Check sheet for the modelled part. Datum: model origin and axes. Units: mm. A direction names the side the tool comes from. Round coordinates to 2 decimals unless told otherwise and drop trailing zeros. Loops run counter-clockwise (first coordinate to the right, second up) from the corner with the lowest first, then second, coordinate; pieces in that order, holes last. Notation, with made-up numbers: M -39,81.5 L 8,81.5 A25 ccw 8,116.5 Z; hole C -32.5,89.5 d7. An arc over 180 degrees is marked long. One line per question, with ' | ' between items. Start each with the question number.
(1) Section check C-C (x = 842). Record the boundary of the cut face in (y, z) (3 decimals).
(2) Section check D-D (y = 13). Record the boundary of the cut face in (x, z) (3 decimals), and give its area (3 significant figures).
(3) Section check B-B (z = -21.5). Record the boundary of the cut face in (x, y).
(4) Draft check along X on faces 3 (the face through (863.31, 22.94, -11.75)), 4 (the face through (847.541, -3.072, -0.905)), 5 (the face through (821.38, 8, 1)). Enter one of: +X half, -X half, draft (parallel to the pull), parting line (faces both ways), or undercut.
(5) Section check A-A (z = -12.7). Record the boundary of the cut face in (x, y), and give its area (3 significant figures).
(6) Go/stop test with flat-tipped pins: P1, Ø15, axis at x = 837, y = 12.5, coming from the -Z side; P2, Ø4, axis at x = 850.5, y = 3, coming from the -Z side. Record where each tip stops, or that it passes through.
(7) Thickness scan on probe 1 along Y at (x, z) = (839, -14.5); probe 2 along Z at (x, y) = (868.5, 13) (3 decimals); probe 3 along Z at (x, y) = (841, 22). Record the ranges inside material, lowest first. Write a range as [from, to].
(8) Tool access check on faces 1 (the face through (831.71, 22.94, -12.56)), 2 (the face through (847.541, 20.468, -0.955)). Record the directions out of +Z, -Z, +X, -X, +Y, -Y that give a thin tool (end or side, any length) a straight path to the whole face; none if there is none.
```python
from build123d import *

# Parameters (mm, degrees)
SKETCH1_W          = 889
SKETCH1_H          = 31.75
EXTRUDE1_DEPTH     = 28.575
EXTRUDE2_REACH     = 891
SKETCH2_W          = 25.4
SKETCH2_H          = 25.4
HOLE1_D            = 6.35
HOLE1_DEPTH        = 3.175
LPATTERN1_COUNT    = 35
LPATTERN1_PITCH    = 25.4
HOLE2_D            = 9.652
HOLE2_DEPTH        = 3.175
LPATTERN2_COUNT    = 12
LPATTERN2_PITCH    = 25.4
HOLE3_D            = 9.652
HOLE3_DEPTH        = 3.175
HOLE4_D            = 9.652
HOLE4_DEPTH        = 3.175
LPATTERN3_COUNT    = 12
LPATTERN3_PITCH    = 25.4
HOLE5_D            = 3.175
HOLE5_DEPTH        = 3.175
HOLE6_D            = 6.35
HOLE6_DEPTH        = 3.175
LPATTERN4_COUNT    = 35
LPATTERN4_PITCH    = 25.4
FILLET1_R          = 3.175
FILLET2_R          = 3.175
FILLET3_R          = 6.35
FILLET4_R          = 6.35
SKETCH16_W         = 145.760071232
SKETCH16_H         = 71.504803879
CUT_EXTRUDE2_DEPTH = 75
SKETCH17_W         = 473.628565651
SKETCH17_H         = 66.908943447
CUT_EXTRUDE3_DEPTH = 186
SKETCH18_W         = 383.094897193
SKETCH18_H         = 93.915816603
CUT_EXTRUDE4_DEPTH = 186
SKETCH19_W         = 44.323760151
SKETCH19_H         = 53.749642994
CUT_EXTRUDE5_DEPTH = 186


with BuildPart() as part:
    # Sketch1 → Extrude1 (new body)
    with BuildSketch(Plane.XY.offset(3.175)):
        with Locations((428.480011997, 8.672957166)):
            Rectangle(SKETCH1_W, SKETCH1_H)
    extrude(amount=-EXTRUDE1_DEPTH)

    # Sketch2 → Extrude2 (cut, up to next)
    with BuildSketch(Plane.ZY.offset(16.019988003), mode=Mode.PRIVATE) as extrude2_sk1:
        with Locations((-12.7, 8.672957166)):
            Rectangle(SKETCH2_W, SKETCH2_H)
    extrude2_tool1 = extrude(extrude2_sk1.sketch, amount=-EXTRUDE2_REACH, mode=Mode.PRIVATE) & part.part
    add(extrude2_tool1.solids().sort_by_distance((-16.019988, 8.672957, -12.7))[0], mode=Mode.SUBTRACT)

    # Hole1
    with Locations(Plane(origin=(0, 24.547957166, 0), x_dir=(-1, 0, 0), z_dir=(0, 1, 0))):
        with Locations((3.319988003, -12.7)):
            hole1 = Hole(HOLE1_D / 2, depth=HOLE1_DEPTH)

    # LPattern1: Hole1 ×35
    with Locations(*[(i * LPATTERN1_PITCH, 0, 0) for i in range(1, LPATTERN1_COUNT)]):
        add(hole1, mode=Mode.SUBTRACT)

    # Hole2
    with Locations(Plane.XY.offset(3.175)):
        with Locations((66.530011997, 10.577957166)):
            hole2 = Hole(HOLE2_D / 2, depth=HOLE2_DEPTH)

    # LPattern2: Hole2 ×12, 8 skipped
    with Locations(*[(i * LPATTERN2_PITCH, 0, 0) for i in range(1, LPATTERN2_COUNT) if i not in (2, 3, 4, 5, 6, 7, 8, 9)]):
        add(hole2, mode=Mode.SUBTRACT)

    # Hole3
    with Locations(Plane.XY.offset(3.175)):
        with Locations((428.480011997, 6.767957166)):
            Hole(HOLE3_D / 2, depth=HOLE3_DEPTH)

    # Hole4
    with Locations(Plane.XY.offset(3.175)):
        with Locations((511.030011997, 10.577957166)):
            hole4 = Hole(HOLE4_D / 2, depth=HOLE4_DEPTH)

    # LPattern3: Hole4 ×12, 8 skipped
    with Locations(*[(i * LPATTERN3_PITCH, 0, 0) for i in range(1, LPATTERN3_COUNT) if i not in (2, 3, 4, 5, 6, 7, 8, 9)]):
        add(hole4, mode=Mode.SUBTRACT)

    # Hole5
    with Locations(Plane.XY.offset(3.175)):
        with Locations((669.780011997, 8.672957166)):
            Hole(HOLE5_D / 2, depth=HOLE5_DEPTH)

    # Hole6
    with Locations(Plane(origin=(0, -4.027042834, 0), x_dir=(-1, 0, 0), z_dir=(0, 1, 0))):
        with Locations((3.319988003, -12.7)):
            hole6 = Hole(HOLE6_D / 2, depth=HOLE6_DEPTH)

    # LPattern4: Hole6 ×35
    with Locations(*[(i * LPATTERN4_PITCH, 0, 0) for i in range(1, LPATTERN4_COUNT)]):
        add(hole6, mode=Mode.SUBTRACT)

    # Fillet1
    fillet1_edges = [part.edges().sort_by_distance(p)[0] for p in [
        (428.480011997, 21.372957166, 0),
    ]]
    fillet(fillet1_edges, radius=FILLET1_R)

    # Fillet2
    fillet2_edges = [part.edges().sort_by_distance(p)[0] for p in [
        (428.480011997, -4.027042834, 0),
    ]]
    fillet(fillet2_edges, radius=FILLET2_R)

    # Fillet3
    fillet3_edges = [part.edges().sort_by_distance(p)[0] for p in [
        (428.480011997, -7.202042834, 3.175),
    ]]
    fillet(fillet3_edges, radius=FILLET3_R)

    # Fillet4
    fillet4_edges = [part.edges().sort_by_distance(p)[0] for p in [
        (428.480011997, 24.547957166, 3.175),
    ]]
    fillet(fillet4_edges, radius=FILLET4_R)

    # Sketch16 → Cut-Extrude2 (cut)
    with BuildSketch(Plane(origin=(0, 24.547957166, 0), x_dir=(1, 0, 0), z_dir=(0, 1, 0))):
        with Locations((40.099976381, -10.352401939)):
            Rectangle(SKETCH16_W, SKETCH16_H)
    extrude(amount=-CUT_EXTRUDE2_DEPTH, mode=Mode.SUBTRACT)

    # Sketch17 → Cut-Extrude3 (cut)
    with BuildSketch(Plane(origin=(0, 24.547957166, 0), x_dir=(1, 0, 0), z_dir=(0, 1, 0))):
        with Locations((288.165729172, -8.054471723)):
            Rectangle(SKETCH17_W, SKETCH17_H)
    extrude(amount=-CUT_EXTRUDE3_DEPTH, mode=Mode.SUBTRACT)

    # Sketch18 → Cut-Extrude4 (cut)
    with BuildSketch(Plane(origin=(0, 24.547957166, 0), x_dir=(1, 0, 0), z_dir=(0, 1, 0))):
        with Locations((621.432563401, -21.557908301)):
            Rectangle(SKETCH18_W, SKETCH18_H)
    extrude(amount=-CUT_EXTRUDE4_DEPTH, mode=Mode.SUBTRACT)

    # Sketch19 → Cut-Extrude5 (cut)
    with BuildSketch(Plane(origin=(0, 24.547957166, 0), x_dir=(1, 0, 0), z_dir=(0, 1, 0))):
        with Locations((799.218131922, -1.474821497)):
            Rectangle(SKETCH19_W, SKETCH19_H)
    extrude(amount=-CUT_EXTRUDE5_DEPTH, mode=Mode.SUBTRACT)


solid = part.part
```
The answers:
1) outline: M -7.202,-25.4 L -4.027,-25.4 L -4.027,-3.175 A3.175 cw -0.852,0 L 18.198,0 A3.175 cw 21.373,-3.175 L 21.373,-25.4 L 24.548,-25.4 L 24.548,-3.175 A6.35 ccw 18.198,3.175 L -0.852,3.175 A6.35 ccw -7.202,-3.175 Z
2) outline: M 821.38,0 L 872.98,0 L 872.98,3.175 L 821.38,3.175 Z | area: 164 mm²
3) outline: M 821.38,-7.2 L 872.98,-7.2 L 872.98,-4.03 L 821.38,-4.03 Z; M 821.38,21.37 L 872.98,21.37 L 872.98,24.55 L 821.38,24.55 Z
4) face 3: undercut | face 4: draft | face 5: -X half
5) outline: M 821.38,-7.2 L 831.71,-7.2 L 831.71,-4.03 L 821.38,-4.03 Z; M 821.38,21.37 L 831.71,21.37 L 831.71,24.55 L 821.38,24.55 Z; M 838.06,-7.2 L 857.11,-7.2 L 857.11,-4.03 L 838.06,-4.03 Z; M 838.06,21.37 L 857.11,21.37 L 857.11,24.55 L 838.06,24.55 Z; M 863.46,-7.2 L 872.98,-7.2 L 872.98,-4.03 L 863.46,-4.03 Z; M 863.46,21.37 L 872.98,21.37 L 872.98,24.55 L 863.46,24.55 Z | area: 247 mm²
6) P1: z = -0.56 | P2: z = 0
7) probe 1: [-7.2, -4.03], [21.37, 24.55] | probe 2: [0, 3.175] | probe 3: [-25.4, 1.91]
8) face 1: +Y, -Y | face 2: -Z, +X, -X
